Autodesk Inventor part; units mm, degrees
ref_plane "YZ Plane" through (0, 0, 0) normal (1, 0, 0) x (0, 1, 0)
ref_plane "XZ Plane" through (0, 0, 0) normal (0, 1, 0) x (-1, 0, 0)
ref_plane "XY Plane" through (0, 0, 0) normal (0, 0, 1) x (1, 0, 0)
sketch "Sketch1" plane through (0, 0, 0) normal (0, 0, 1) x (1, 0, 0)
  line L0 (0, 0) -> (46, 0)
  line L1 (46, 0) -> (46, 20)
  line L2 (46, 20) -> (0, 20)
  line L3 (0, 20) -> (0, 0)
  line L4 (0, 0) -> (-46, 0)
  line L5 (-46, 0) -> (-46, -20)
  line L6 (-46, -20) -> (0, -20)
  line L7 (0, -20) -> (0, 0)
  line L8 (-46, -20) -> (46, -20)
  line L9 (46, -20) -> (46, 20)
  line L10 (46, 20) -> (-46, 20)
  line L11 (-46, 20) -> (-46, -20)
  point P0 (0, 20)
  point P1 (0, -20)
  dimension "d7" = 40
  dimension "d8" = 92
extrude "Extrusion1" add sketch "Sketch1" along normal blind 8
sketch "Sketch2" plane through (0, 0, 0) normal (0, 0, -1) x (-1, 0, 0)
  circle A0 centre (24, 16) radius 1.25 construction
  circle A1 centre (-33, 16.5) radius 1.5
  circle A2 centre (-14, 16) radius 1.25 construction
  circle A3 centre (14, 16) radius 1.25 construction
  circle A4 centre (4.5, 16.5) radius 1.5
  circle A5 centre (-5, -16.5) radius 1.5
  circle A6 centre (32.5, -16.5) radius 1.5
  point P0 (0, 0)
extrude "Extrusion2" cut sketch "Sketch2" against normal through all
properties part number "Bottom"
CAD build for the part. Positions are in the model's coordinates, mm. Round coordinates to 2 decimals unless told otherwise and drop trailing zeros. Loops run counter-clockwise (first coordinate to the right, second up) from the corner with the lowest first, then second, coordinate; pieces in that order, holes last. Notation, with made-up numbers: M 62,40 L 101,40 A25 ccw 101,54 Z; hole C -3.5,77.5 d9. An arc over 180 degrees is marked long. One line per question, with ' | ' between items. Start each with the question number.
Item 1: Cut at B-B, the plane y = 16.5. Write the cut outline in (x, z), plus the area to 3 significant figures.
Item 2: Wall check: line 1 (Y direction, x = -32.5, z = 2.5); line 2 (Y direction, x = -5.5, z = 5.25). Give the ranges that are in metal, low to high.
Item 3: Cut at A-A, the plane x = -32.5. Write the cut outline in (y, z).
Item 4: Two-plate mould, pull along Y, no slides. Class faces 1 (the cylindrical face through (6.5, -16.43, 3.94)), 2 (the flat face through (1, 20, 4)), 3 (the flat face through (-1, 0, 8)): pulls with the +Y half, pulls with the -Y half, needs draft (parallel to the pull), parting line crosses it, or undercut.
Item 5: Pin check, flat tip, straight feed: pin 1 Ø2.5 at (x, y) = (5, -16.5) entering from +Z. Stop position of the tip, or through.
Responses:
1) outline: M -46,0 L -6,0 L -6,8 L -46,8 Z; M -3,0 L 31.5,0 L 31.5,8 L -3,8 Z; M 34.5,0 L 46,0 L 46,8 L 34.5,8 Z | area: 688 mm²
2) line 1: y = -20 to -18, -15 to 20 | line 2: y = -20 to 15.38, 17.62 to 20
3) outline: M -20,0 L -18,0 L -18,8 L -20,8 Z; M -15,0 L 20,0 L 20,8 L -15,8 Z
4) face 1: undercut | face 2: pulls with the +Y half | face 3: needs draft
5) pin 1: passes through
